Can you work these out from the drawing? Everything is in mm from the part's minimum corner. A direction names the side the tool comes from. Coordinates: 2 decimals unless noted, no trailing zeros. Loops run counter-clockwise (first coordinate to the right, second up) from the corner with the lowest first, then second, coordinate; pieces in that order, holes last. Notation, with made-up numbers: (39.25, -39.5) -> (45.25, -39.5) arc R11 ccw to (45.25, -34.5) -> close; hole circle Ø6 at (69.25, 1.5). An arc over 180 degrees is marked (long way). Put each result on its own line as item: value. Start each with the question number.
Item 1: For the marked faces 5 and 6, which set-ups out of +Z, -Z, +X, -X, +Y, -Y let a thin tool reach every point of the face, with its end or its side?
Item 2: If we section it at B-B on y = 6.5: Please give me the cut outline in (x, z) (3 decimals).
Item 3: If we section it at C-C on x = 16: Please give me the cut outline in (y, z) (3 decimals).
Item 4: Will this pin go through, and if not, where does the flat tip stop? P1, Ø4, axis at y = 19.05, z = 12.7, coming from the +X side.
Item 5: Please list where these lines run through material, in increasing order: L1, parallel to Y at x = 6.75, z = 8 (3 decimals); L2, parallel to X at y = 10, z = 31.5 (3 decimals); L3, parallel to Y at x = 1, z = 63.5 (3 decimals). Write a range as from..to.
Item 6: If we section it at A-A on z = 63.5: Please give me the cut outline in (x, y) (3 decimals), plus the area to 3 significant figures.
Item 7: We'd pull the mould along Y, two halves only. Please class the marked faces 1, 2, 3 and 4: pulls with the +Y half, pulls with the -Y half, needs draft (parallel to the pull), parting line crosses it, or undercut.
Item 8: If we section it at D-D on y = 19.05: State how many separate pieces and enclosed holes the cut face has, plus the area to 3 significant figures.
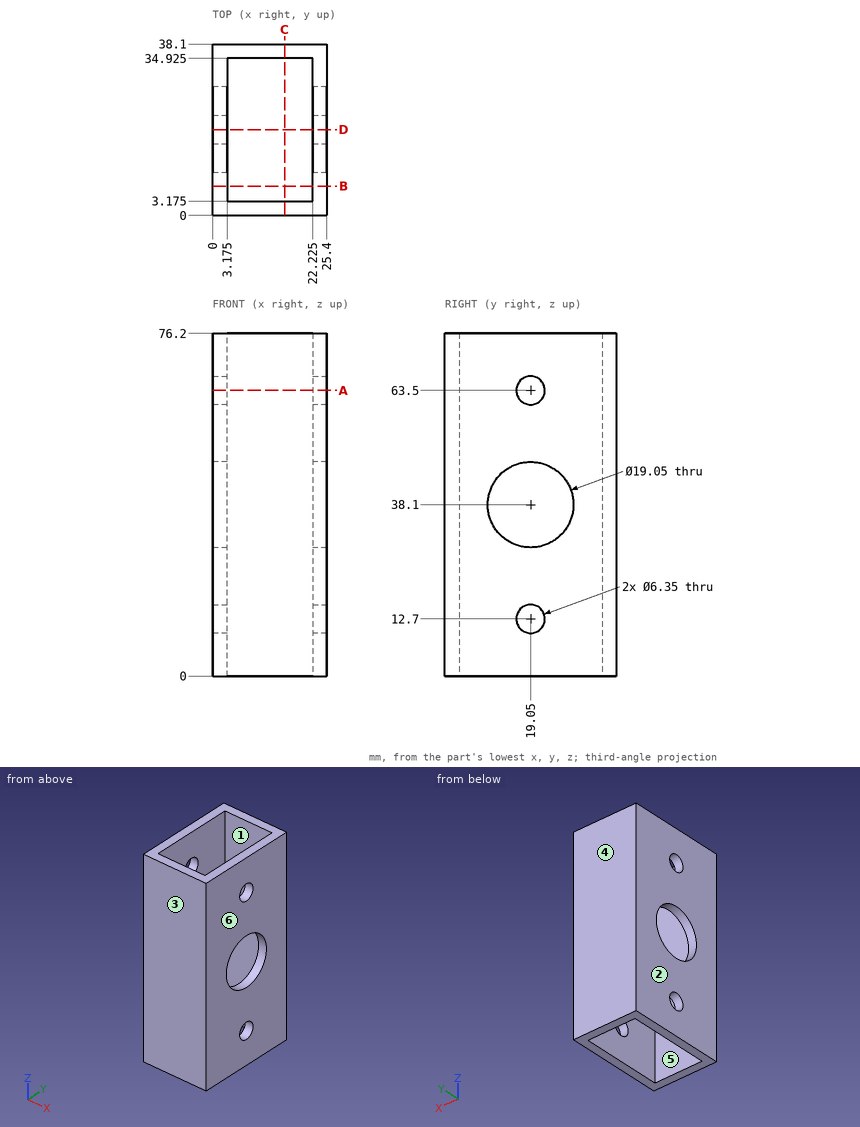
Solutions:
1. face 5: +Z, -Z
1. face 6: +Z, -Z, +X, +Y, -Y
2. outline: (0, 0) -> (3.175, 0) -> (3.175, 76.2) -> (0, 76.2) -> close; (22.225, 0) -> (25.4, 0) -> (25.4, 76.2) -> (22.225, 76.2) -> close
3. outline: (0, 0) -> (3.175, 0) -> (3.175, 76.2) -> (0, 76.2) -> close; (34.925, 0) -> (38.1, 0) -> (38.1, 76.2) -> (34.925, 76.2) -> close
4. P1: through
5. L1: 0..3.175, 34.925..38.1
5. L2: 0..3.175, 22.225..25.4
5. L3: 0..15.875, 22.225..38.1
6. outline: (0, 0) -> (25.4, 0) -> (25.4, 15.875) -> (22.225, 15.875) -> (22.225, 3.175) -> (3.175, 3.175) -> (3.175, 15.875) -> (0, 15.875) -> close; (0, 22.225) -> (3.175, 22.225) -> (3.175, 34.925) -> (22.225, 34.925) -> (22.225, 22.225) -> (25.4, 22.225) -> (25.4, 38.1) -> (0, 38.1) -> close
6. area: 323 mm^2
7. face 1: undercut
7. face 2: needs draft
7. face 3: pulls with the -Y half
7. face 4: pulls with the +Y half
8. separate pieces: 8
8. enclosed holes: 0
8. area: 282 mm^2
